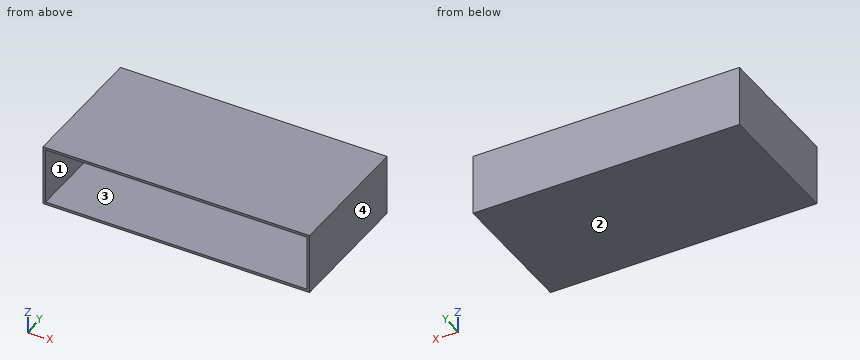
```python
from build123d import *

# Parameters (mm, degrees)
F0_W     = 1020
F0_H     = 233
F0_W_2   = 1000
F0_H_2   = 213
F1_DEPTH = 509
F2_W     = 1020
F2_H     = 233
F2_W_2   = 1000
F2_H_2   = 213
F3_DEPTH = 10


with BuildPart() as f1:
    # F0 (on Front) → F1 (new body)
    with BuildSketch(Plane.XZ):
        with Locations((0, 106.5)):
            Rectangle(F0_W, F0_H)
        with Locations((0, 106.5)):
            Rectangle(F0_W_2, F0_H_2, mode=Mode.SUBTRACT)
    extrude(amount=-F1_DEPTH)

    # F2 (on face) → F3 (join)
    with BuildSketch(Plane(origin=(0, 509, 0), x_dir=(-1, 0, 0), z_dir=(0, 1, 0))):
        with Locations((0, 106.5)):
            Rectangle(F2_W, F2_H)
        with Locations((0, 106.5)):
            Rectangle(F2_W_2, F2_H_2, mode=Mode.SUBTRACT)
        with Locations((0, 106.5)):
            Rectangle(F2_W_2, F2_H_2)
    extrude(amount=F3_DEPTH)


solid = f1.part
```
Can you work these out from the model? Positions are in its coordinate system, mm. Face numbers are marked on the shaded views. Coordinates: 2 decimals unless noted, no trailing zeros. Order: outer loops, then holes, each group sorted by start corner. A loop starts at its lowest first (then second) coordinate and runs counter-clockwise, first axis right, second up.
1. If we section it at C-C (x = -229): Please give me the cut outline in (y, z), then the cut area to 3 significant figures.
2. Thinking about a two-plate mould opening in X: for the marked faces 1, 2, 3 and 4, which applies, +X half, -X half, draft (parallel to the pull), parting line (faces both ways), or undercut?
3. If we section it at A-A (y = 323): Please give me the cut outline in (x, z), then the cut area to 3 significant figures.
4. I need wall thicknesses on line 1 (X direction, y = 277.5, z = 75); line 2 (Z direction, x = -188.5, y = 431); line 3 (Y direction, x = -276, z = 184.5). Which ranges of each line are inside material? Lowest first, please.
5. If we section it at B-B (z = 85): Please give me the cut outline in (x, y), then the cut area to 3 significant figures.
6. I'm going to push a flat-ended pin straight in: pin 1 (8 mm diameter, centred on x = 244.5, z = 67.5, fed in from -Y). Where does the tip first touch, or does it pass through?
Entries:
1. outline: (0, -10) - (519, -10) - (519, 223) - (0, 223) - (0, 213) - (509, 213) - (509, 0) - (0, 0) - close
1. area: 12,500 mm2
2. face 1: undercut
2. face 2: draft
2. face 3: undercut
2. face 4: +X half
3. outline: (-510, -10) - (510, -10) - (510, 223) - (-510, 223) - close; hole (-500, 0) - (500, 0) - (500, 213) - (-500, 213) - close
3. area: 24,700 mm2
4. line 1: x = -510 to -500, 500 to 510
4. line 2: z = -10 to 0, 213 to 223
4. line 3: y = 509 to 519
5. outline: (-510, 0) - (-500, 0) - (-500, 509) - (500, 509) - (500, 0) - (510, 0) - (510, 519) - (-510, 519) - close
5. area: 20,400 mm2
6. pin 1: stops at y = 509
